For this review, take the finished solid that the model builds, in its own axes (mm). A direction names the side the tool comes from. Round coordinates to 2 decimals unless told otherwise and drop trailing zeros. Write each loop counter-clockwise with the first axis right and the second up, starting at its lowest first coordinate (ties: lowest second). Pieces come first, ordered by that corner, then holes. Notation, with made-up numbers: (0.5, -35.75) - (52.5, -35.75) arc R20 ccw to (52.5, -27.75) - close; hole circle Ø9 at (86.5, 6.5). An arc over 180 degrees is marked (long way). Answer in a Markdown table with one row per item. Add a question column.
Autodesk Inventor part; units mm, degrees
ref_plane "YZ Plane" through (0, 0, 0) normal (1, 0, 0) x (0, 1, 0)
ref_plane "XZ Plane" through (0, 0, 0) normal (0, 1, 0) x (-1, 0, 0)
ref_plane "XY Plane" through (0, 0, 0) normal (0, 0, 1) x (1, 0, 0)
sketch "Sketch1" plane through (0, 0, 0) normal (1, 0, 0) x (0, 1, 0)
  circle A0 centre (0, 0) radius 4.75
  line L0 (10, 45) -> (-10, 45)
  line L1 (10, 38) -> (-10, 38)
  line L2 (10, 45) -> (10, 38)
  line L3 (-10, 38) -> (-10, 45)
  line L4 (-4.75, 0) -> (-8.4137, 0)
  line L5 (-14, 0) -> (14, 0)
  line L6 (10, -55) -> (-10, -55)
  line L7 (-10, -55) -> (-10, -48)
  line L8 (-10, -48) -> (10, -48)
  line L9 (10, -48) -> (10, -55)
  line L10 (10, 38) -> (10, -48)
  line L11 (-10, -48) -> (-10, 38)
  point P0 (0, 45)
  point P1 (0, -55)
  dimension "d0" = 9.5
  dimension "d1" = 20
  dimension "d2" = 0
  dimension "d3" = 7
  dimension "d4" = 45
  dimension "d8" = 20
  dimension "d9" = 7
  dimension "d10" = 0
  dimension "d11" = 55
extrude "Extrusion1" add sketch "Sketch1" along normal blind 10 contours L5 L10 L8 L11 L4 A0 | A0 L4 L5 L11 L1 L10 | L1 L3 L0 L2 | L9 L6 L7 L8
sketch "Sketch2" plane through (0, -10, -55) normal (0, 0, -1) x (-1, 0, 0)
  circle A0 centre (-5, 10) radius 2.475
  point P0 (0, 10)
  dimension "d12" = 4.95
extrude "Extrusion2" add sketch "Sketch2" along normal blind 4.9
chamfer "Chamfer1" distance 0.5 angle 45 1 edges at (7.475, 0, -59.9)
sketch "Sketch3" plane through (0, -10, -55) normal (0, 0, -1) x (-1, 0, 0)
  circle A0 centre (-5, 10) radius 2.475
  circle A1 centre (-5, 10) radius 7
  circle A2 centre (-5, 10) radius 17.4724
  point P0 (0, 10)
  dimension "d18" = 14
extrude "Extrusion3" cut sketch "Sketch3" against normal through all contours A2
sketch "Sketch4" plane through (0, 0, 0) normal (1, 0, 0) x (0, 1, 0)
  circle A0 centre (0, 0) radius 7.5
  circle A1 centre (0, 0) radius 12.5
  dimension "d21" = 15
  dimension "d22" = 5
extrude "Extrusion4" add sketch "Sketch4" along normal up to surface (10 mm away)
extrude "Extrusion5" cut sketch "Sketch4" along normal blind 10 contours A0
properties part number "nozzle holder v1"
Q1. Add section A-A on y = 0. State the section outline as (x, z) points (3 decimals), then the cut area to 3 significant figures.
Q2. Add section B-B on z = 0. State the section outline as (x, y) points.
Q3. Add section D-D on z = 28.5. State the section outline as (x, y) points.
Q4. Add section C-C on x = 8.5. State the section outline as (y, z) points.
Q5. Insertion check: pin 1 Ø1.5 at (x, y) = (2.5, -7) entering from -Z; pin 2 Ø6 at (y, z) = (1.5, 0.5) entering from +X; pin 3 Ø1 at (y, z) = (-6, -17) entering from -X; pin 4 Ø1.5 at (y, z) = (1, -41.5) entering from -X. Each pin has a flat end and moves straight along its axis. Give the tip position at first contact, or say it passes through.
Q6. Tool access review of faces 1 (the face through (2.64, -0.74, -57.17)), 2 (the face through (5, -7, 27)), 3 (the face through (5, 7, -33)), 4 (the face through (5, 7, 27)): name each direction out of +Z, -Z, +X, -X, +Y, -Y from which nothing blocks a thin tool from reaching the whole face with its end or side.
Q7. To check wall thickness, follow probe 1 along Z at (x, y) = (9.5, 0.5); probe 2 along Z at (x, y) = (6, 0); probe 3 along Y at (x, z) = (3, 0). State the ranges of each line that lie inside material, in increasing order.
Answer sheet:
| question | item | result |
|---|---|---|
| 1 | outline | (0, -55) - (2.525, -55) - (2.525, -59.4) - (3.025, -59.9) - (6.975, -59.9) - (7.475, -59.4) - (7.475, -55) - (10, -55) - (10, -7.5) - (0, -7.5) - close; (0, 7.5) - (10, 7.5) - (10, 45) - (0, 45) - close |
| 1 | area | 874 mm² |
| 2 | outline | (0, -12.5) - (10, -12.5) - (10, -7.5) - (0, -7.5) - close; (0, 7.5) - (10, 7.5) - (10, 12.5) - (0, 12.5) - close |
| 3 | outline | (0, -4.9) arc R7 ccw to (10, -4.9) - (10, 4.9) arc R7 ccw to (0, 4.9) - close |
| 4 | outline | (-6.06, -55) - (6.06, -55) - (6.06, -10.93) arc R12.5 ccw to (6.06, 10.93) - (6.06, 45) - (-6.06, 45) - (-6.06, 10.93) arc R12.5 ccw to (-6.06, -10.93) - close; hole circle Ø15 at (0, 0) |
| 5 | pin 1 | stops at z = -55 |
| 5 | pin 2 | passes through |
| 5 | pin 3 | stops at x = 0.67 |
| 5 | pin 4 | stops at x = 0 |
| 6 | face 1 | -Z |
| 6 | face 2 | +Z, -Y |
| 6 | face 3 | -Z, +Y |
| 6 | face 4 | +Z, +Y |
| 7 | probe 1 | z = -55 to -7.48, 7.48 to 45 |
| 7 | probe 2 | z = -59.9 to -7.5, 7.5 to 45 |
| 7 | probe 3 | y = -12.5 to -7.5, 7.5 to 12.5 |
